Work out the finished part from the listing and answer in its coordinate system (mm). Face numbers are marked on the shaded views. A direction names the side the tool comes from. Round coordinates to 2 decimals unless told otherwise and drop trailing zeros. Loops run counter-clockwise (first coordinate to the right, second up) from the corner with the lowest first, then second, coordinate; pieces in that order, holes last. Notation, with made-up numbers: (69.25, -30) - (99.25, -30) arc R24 ccw to (99.25, -15) - close; hole circle Ø2 at (27.25, 83). An arc over 180 degrees is marked (long way). Return JSON: item names as keys, results as strings.
from build123d import *

# Parameters (mm, degrees)
F2_R     = 1.99999
F4_DEPTH = 3


# Not quite as in the source:
# - a fillet or chamfer is up to 0.001 mm smaller than in the source, because OpenCascade refuses the exact size
# - a feature names something its author has since deleted; it is built from what else it names


with BuildPart() as f1:
    # F0 (on Front) → F1 (revolve)
    with BuildSketch(Plane.XZ):
        Polygon((2.5, 2), (3.5, 2), (3.5, 0), (7.5, 0), (7.5, 5), (9.5, 5), (9.5, 10), (2.5, 10), align=None)
    revolve(axis=Axis((0, 0, 8.8058942929), (0, 0, 1)))

    # F2 (radius 2 in the source; OpenCascade refuses exactly that, so slightly less here)
    f2_edges = [f1.edges().sort_by_distance(p)[0] for p in [
        (-9.5, 0, 5),
    ]]
    fillet(f2_edges, radius=F2_R)

    # F3 (on face) → F4 (cut)
    with BuildSketch(Plane(origin=(0, 0, 0), x_dir=(1, 0, 0), z_dir=(0, 0, -1))):
        with BuildLine():
            ThreePointArc((-1.75, 3.0310889132), (0.8206712512, 3.402425414), (2.9393876913, 1.9))
            Line((2.9393876913, 1.9), (2.9393876913, 6.9))
            ThreePointArc((2.9393876913, 6.9), (-0.4530350492, 7.486304779), (-3.75, 6.4951905284))
            Line((-3.75, 6.4951905284), (-1.75, 3.0310889132))
        make_face()
    extrude(amount=-F4_DEPTH, mode=Mode.SUBTRACT)


solid = f1.part
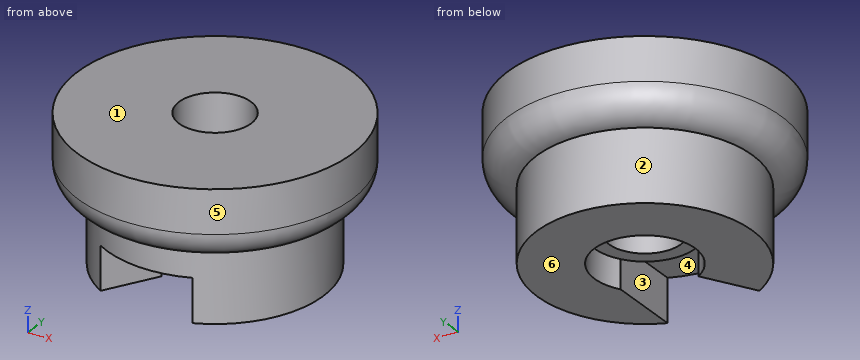
1) Section C-C (z = 9) is taken. Give the vertices of the cut face in (x, y), and give its area (3 significant figures).
Verdict:
{"outline": "circle Ø19 at (0, 0); hole circle Ø5 at (0, 0)", "area": "264 mm2"}
2) Find the intervals of material crossed by L1, parallel to X at y = 0, z = 1.1; L2, parallel to Y at x = 0, z = 3.5; L3, parallel to X at y = -3.5, z = 1, in increasing order.
Verdict:
{"L1": "x = -7.5 to -3.5, 3.5 to 7.5", "L2": "y = -7.5 to -2.5, 2.5 to 7.5", "L3": "x = -6.63 to -2.02, 2.94 to 6.63"}
3) Flat-ended cylindrical pins translate along their axes: pin 1 (4.5 mm diameter, centred on x = -1.5, y = -4, fed in from -Z); pin 2 (2.5 mm diameter, centred on y = -4, z = 1, fed in from -X); pin 3 (3 mm diameter, centred on x = -5.5, z = 3, fed in from +Y); pin 4 (1.5 mm diameter, centred on x = -4, z = 5, fed in from +Y). Find the tip coordinate at first contact, or state that the pin passes through.
Verdict:
{"pin 1": "stops at z = 0", "pin 2": "stops at x = -6.98", "pin 3": "stops at y = 6.34", "pin 4": "stops at y = 8.21"}
4) A tool of negligible diameter and unlimited length cuts with its end or side. For the marked faces 1, 2 and 3, from which of +Z, -Z, +X, -X, +Y, -Y can it reach the whole face along a straight path? Write none if from no direction.
Verdict:
{"face 1": "+Z, +X, -X, +Y, -Y", "face 2": "-Z", "face 3": "-Z, -Y"}
5) Determine the mould class of the marked faces 4, 5 and 6 for opening direction X: pulls with the +X half, pulls with the -X half, needs draft (parallel to the pull), parting line crosses it, or undercut.
Verdict:
{"face 4": "undercut", "face 5": "parting line crosses it", "face 6": "needs draft"}
6) Section D-D (z = 4.5) is taken. Give the vertices of the cut face in (x, y).
Verdict:
{"outline": "circle Ø15 at (0, 0); hole circle Ø5 at (0, 0)"}
